The model under review builds one solid part; all positions refer to its coordinate system, in mm. Coordinates: 2 decimals unless noted, no trailing zeros. Loops run counter-clockwise (first coordinate to the right, second up) from the corner with the lowest first, then second, coordinate; pieces in that order, holes last. Notation, with made-up numbers: M 35,14 L 67,14 A20 ccw 67,22 Z; hole C -30,80.5 d11. An arc over 180 degrees is marked long. Use one line per item in the form item = value.
Autodesk Inventor part; units mm, degrees
ref_plane "Work Plane1" through (0, 0, 0) normal (0, 0, 1) x (1, 0, 0)
ref_plane "YZ Plane" through (0, 0, 0) normal (1, 0, 0) x (0, 1, 0)
ref_plane "XZ Plane" through (0, 0, 0) normal (0, 1, 0) x (-1, 0, 0)
ref_plane "Work Plane1" through (0, 0, 0) normal (0, 0, 1) x (1, 0, 0)
sketch "Sketch1" plane through (0, 0, 0) normal (0, 0, 1) x (1, 0, 0)
  arc A0 (16.9393, 20.5607) -> (15.8787, 21) centre (15.8787, 19.5) ccw
  line L0 (15.8787, 21) -> (-15.8787, 21)
  arc A1 (-15.8787, 21) -> (-16.9393, 20.5607) centre (-15.8787, 19.5) ccw
  line L1 (-16.9393, 20.5607) -> (-20.5607, 16.9393)
  arc A2 (-20.5607, 16.9393) -> (-21, 15.8787) centre (-19.5, 15.8787) ccw
  line L2 (-21, 15.8787) -> (-21, -15.8787)
  arc A3 (-21, -15.8787) -> (-20.5607, -16.9393) centre (-19.5, -15.8787) ccw
  line L3 (-20.5607, -16.9393) -> (-16.9393, -20.5607)
  arc A4 (-16.9393, -20.5607) -> (-15.8787, -21) centre (-15.8787, -19.5) ccw
  line L4 (-15.8787, -21) -> (15.8787, -21)
  arc A5 (15.8787, -21) -> (16.9393, -20.5607) centre (15.8787, -19.5) ccw
  line L5 (16.9393, -20.5607) -> (20.5607, -16.9393)
  arc A6 (20.5607, -16.9393) -> (21, -15.8787) centre (19.5, -15.8787) ccw
  line L6 (21, -15.8787) -> (21, 15.8787)
  arc A7 (21, 15.8787) -> (20.5607, 16.9393) centre (19.5, 15.8787) ccw
  line L7 (20.5607, 16.9393) -> (16.9393, 20.5607)
  circle A8 centre (-15.5, -15.5) radius 1.5
  circle A9 centre (-15.5, 15.5) radius 1.5
  circle A10 centre (15.5, -15.5) radius 1.5
  circle A11 centre (15.5, 15.5) radius 1.5
  circle A12 centre (0, 0) radius 11.2
  circle A13 centre (-15.5, 15.5) radius 2
  circle A14 centre (-15.5, -15.5) radius 2
  circle A15 centre (15.5, -15.5) radius 2
  circle A16 centre (15.5, 15.5) radius 2
  point P0 (0, 0)
  dimension "d0" = 4
  dimension "d1" = 4
  dimension "d2" = 4
  dimension "d3" = 4
extrude "Extrusion1" add sketch "Sketch1" along normal blind 3 contours L7 A7 L6 A6 L5 A5 L4 A4 L3 A3 L2 A2 L1 A1 L0 A0
properties part number "Part2_3DPrint"
1. Wall thickness on line 1 along Y through (x, z) = (-15.5, 1.25); line 2 along Y through (x, z) = (14, 1.35); line 3 along Y through (x, z) = (0, 1.9): over which ranges is each line inside the solid? List them lowest first. Write a range as from..to.
Response values:
line_1 = -21..-17.5, -13.5..13.5, 17.5..21
line_2 = -21..-16.82, -14.18..14.18, 16.82..21
line_3 = -21..-11.2, 11.2..21
2. The part is to be moulded in two halves that separate along X. For faces 1 (the face through (-16.445, -20.889, 1.479)), 2 (the face through (20.889, -16.445, 1.479)), 3 (the face through (15.24, -17.483, 1.479)), say which applies: pulls with the +X half, pulls with the -X half, needs draft (parallel to the pull), parting line crosses it, or undercut.
Response values:
face_1 = pulls with the -X half
face_2 = pulls with the +X half
face_3 = undercut
3. Add section C-C (x = -8). State the section outline as (y, z) points, then the cut area to 3 significant figures.
Response values:
outline = M -21,0 L -7.84,0 L -7.84,3 L -21,3 Z; M 7.84,0 L 21,0 L 21,3 L 7.84,3 Z
area = 79.0 mm^2
4. Add section B-B (y = 0). State the section outline as (x, z) points.
Response values:
outline = M -21,0 L -11.2,0 L -11.2,3 L -21,3 Z; M 11.2,0 L 21,0 L 21,3 L 11.2,3 Z
5. Add section A-A (z = 2.2). State the section outline as (x, y) points, then the cut area to 3 significant figures.
Response values:
outline = M -21,-15.88 A1.5 ccw -20.56,-16.94 L -16.94,-20.56 A1.5 ccw -15.88,-21 L 15.88,-21 A1.5 ccw 16.94,-20.56 L 20.56,-16.94 A1.5 ccw 21,-15.88 L 21,15.88 A1.5 ccw 20.56,16.94 L 16.94,20.56 A1.5 ccw 15.88,21 L -15.88,21 A1.5 ccw -16.94,20.56 L -20.56,16.94 A1.5 ccw -21,15.88 Z; hole C -15.5,-15.5 d4; hole C -15.5,15.5 d4; hole C 0,0 d22.4; hole C 15.5,-15.5 d4; hole C 15.5,15.5 d4
area = 1,280 mm^2
6. Insertion check: P1, Ø1.5, axis at x = 8, y = 7, coming from the -Z side. The pin has a flat end and moves straight along its axis. Give the tip position at first contact, or say it passes through.
Response values:
P1 = 0
